from build123d import *

# Parameters (mm, degrees)
F2_DEPTH = 5
F1_R     = 1.5
F3_DEPTH = 5


with BuildPart() as f2:
    # F0 (on Top) → F2 (new body)
    with BuildSketch(Plane.XY):
        with BuildLine():
            add(Edge.make_bspline(
                [(28.7786647677, 16.4962057024), (27.3534332712, 16.4962057024), (25.9282017748, 16.3979139179), (24.5029702783, 16.3979139179)],
                knots=[0, 0, 0, 0, 4.2768241304, 4.2768241304, 4.2768241304, 4.2768241304], degree=3))
            add(Edge.make_bspline(
                [(28.7786647677, 16.4962057024), (30.1958868901, 16.5288864324), (31.6131090124, 16.5615671625), (33.0303311348, 16.5942478925)],
                knots=[0, 0, 0, 0, 4.252796629, 4.252796629, 4.252796629, 4.252796629], degree=3))
            add(Edge.make_bspline(
                [(34.0554304421, 15.8441737294), (33.7053959568, 16.1608718336), (33.3803656201, 16.2775497884), (33.0303311348, 16.5942478925)],
                knots=[0, 0, 0, 0, 1.2702125176, 1.2702125176, 1.2702125176, 1.2702125176], degree=3))
            add(Edge.make_bspline(
                [(35.030528903, 7.8683812171), (34.7054960827, 10.5269787212), (34.3804632624, 13.1855762253), (34.0554304421, 15.8441737294)],
                knots=[0, 0, 0, 0, 8.0351778579, 8.0351778579, 8.0351778579, 8.0351778579], degree=3))
            add(Edge.make_bspline(
                [(36.1056365073, 5.4181381129), (35.9264295305, 5.3620166626), (35.3451776861, 5.1799886127), (35.15918074, 6.7691662645), (35.030528903, 7.8683812171)],
                knots=[0, 0, 0, 0, 0.3083121001, 1, 1, 1, 1], degree=3))
            add(Edge.make_bspline(
                [(38.8059057295, 8.4184361622), (37.4535769802, 6.9203687349), (36.1012482309, 5.4223013077), (36.1056365073, 5.4181381129)],
                knots=[0, 0, 0, 0, 0.9144176852, 0.9144176852, 0.9144176852, 0.9144176852], degree=3))
            add(Edge.make_bspline(
                [(39.8560129106, 14.1940098256), (39.2937416175, 11.3257224468), (38.7314703243, 8.4574350679), (38.8059057295, 8.4184361622)],
                knots=[0, 0, 0, 0, 0.9279806118, 0.9279806118, 0.9279806118, 0.9279806118], degree=3))
            add(Edge.make_bspline(
                [(43.4063635767, 19.4445308298), (41.6661026772, 16.796114764), (39.8167199055, 13.9816315759), (39.8538236249, 14.1821767609), (39.8560129106, 14.1940098256)],
                knots=[0, 0, 0, 0, 0.9409955181, 1, 1, 1, 1], degree=3))
            add(Edge.make_bspline(
                [(46.1316332221, 30.1705934107), (46.201065216, 26.0141822855), (46.2669693032, 19.7845163706), (44.1314354539, 19.7195578367), (43.4063635767, 19.4445308298)],
                knots=[0, 0, 0, 0, 0.6856364339, 1, 1, 1, 1], degree=3))
            add(Edge.make_bspline(
                [(44.0814308822, 39.2214953899), (44.942471716, 37.026856873), (45.9936424251, 33.4912353698), (46.1571893395, 30.7073156698), (46.1316332221, 30.1705934107)],
                knots=[0, 0, 0, 0, 0.5973818248, 1, 1, 1, 1], degree=3))
            add(Edge.make_bspline(
                [(37.9308201373, 46.5972237289), (39.7218772443, 45.1967775697), (42.7448053753, 42.833118659), (43.922661607, 39.3325250293), (44.0814308822, 39.2214953899)],
                knots=[0, 0, 0, 0, 0.5634229372, 0.9509395541, 0.9509395541, 0.9509395541, 0.9509395541], degree=3))
            add(Edge.make_bspline(
                [(28.3798743039, 49.4475066662), (30.3463351664, 49.2764352977), (34.0485912428, 48.954359214), (36.6916346322, 47.3496080436), (37.9308201373, 46.5972237289)],
                knots=[0, 0, 0, 0, 0.5311520386, 1, 1, 1, 1], degree=3))
            add(Edge.make_bspline(
                [(20.4540863633, 47.2972951829), (21.8867810289, 47.9304252414), (24.6135730188, 49.1354370372), (27.1677144968, 49.3470690664), (28.3798743039, 49.4475066662)],
                knots=[0, 0, 0, 0, 0.5254139923, 1, 1, 1, 1], degree=3))
            add(Edge.make_bspline(
                [(12.128260918, 36.621235311), (13.2656434176, 39.1604577253), (15.3840794859, 43.8898960188), (18.8493227012, 46.2187817818), (20.4540863633, 47.2972951829)],
                knots=[0, 0, 0, 0, 0.5368972501, 1, 1, 1, 1], degree=3))
            add(Edge.make_bspline(
                [(11.1531633884, 25.0700879842), (11.0426565419, 27.5454372876), (10.8424476096, 32.0301100206), (11.730414239, 35.2006838689), (12.128260918, 36.621235311)],
                knots=[0, 0, 0, 0, 0.5519576234, 1, 1, 1, 1], degree=3))
            add(Edge.make_bspline(
                [(12.128260918, 20.2196072787), (11.9396298399, 20.7302181813), (11.4960442281, 21.93097286), (11.2783087006, 23.9243676733), (11.1531633884, 25.0700879842)],
                knots=[0, 0, 0, 0, 0.4252416515, 1, 1, 1, 1], degree=3))
            add(Edge.make_bspline(
                [(14.2806209624, 19.1009379923), (13.5631676142, 19.4738277545), (12.8457142661, 19.8467175166), (12.128260918, 20.2196072787)],
                knots=[0, 0, 0, 0, 2.4257111809, 2.4257111809, 2.4257111809, 2.4257111809], degree=3))
            add(Edge.make_bspline(
                [(17.6962614059, 13.7686077505), (16.5577145914, 15.5460511645), (15.4191677769, 17.3234945784), (14.2806209624, 19.1009379923)],
                knots=[0, 0, 0, 0, 6.3324833555, 6.3324833555, 6.3324833555, 6.3324833555], degree=3))
            add(Edge.make_bspline(
                [(18.826616928, 7.7482336201), (18.449831754, 9.7550249969), (18.07304658, 11.7618163737), (17.6962614059, 13.7686077505)],
                knots=[0, 0, 0, 0, 6.1255700369, 6.1255700369, 6.1255700369, 6.1255700369], degree=3))
            add(Edge.make_bspline(
                [(21.8245182186, 5.4629491642), (21.7108202341, 5.3376502894), (21.4165861788, 5.0133947963), (20.4957638936, 6.0671498654), (19.4532904711, 7.1170784645), (18.826616928, 7.7482336201)],
                knots=[0, 0, 0, 0, 0.2007630192, 0.5195458611, 1, 1, 1, 1], degree=3))
            add(Edge.make_bspline(
                [(22.9794476181, 12.7365430817), (22.5944711516, 10.3120117759), (22.2094946851, 7.88748047), (21.8245182186, 5.4629491642)],
                knots=[0, 0, 0, 0, 7.3647152283, 7.3647152283, 7.3647152283, 7.3647152283], degree=3))
            add(Edge.make_bspline(
                [(24.5029702783, 16.3979139179), (24.2545480757, 16.457738394), (23.7733196994, 16.5750358032), (23.1531511766, 15.0702995523), (23.0738569515, 13.5969865217), (22.9794476181, 12.7365430817)],
                knots=[0, 0, 0, 0, 0.2229298737, 0.552268584, 1, 1, 1, 1], degree=3))
        make_face()
        with BuildLine():
            add(Edge.make_bspline(
                [(19.7707619518, 25.4675038159), (20.2849085132, 25.757982706), (20.6410096337, 26.1077272395), (21.1551561952, 26.3982061297)],
                knots=[0, 0, 0, 0, 1.6681589307, 1.6681589307, 1.6681589307, 1.6681589307], degree=3))
            add(Edge.make_bspline(
                [(21.1551561952, 26.3982061297), (21.8123979867, 26.8640990059), (22.4696397781, 27.329991882), (23.1268815696, 27.7958847582)],
                knots=[0, 0, 0, 0, 2.4168588087, 2.4168588087, 2.4168588087, 2.4168588087], degree=3))
            add(Edge.make_bspline(
                [(23.1268815696, 27.7958847582), (23.4302642999, 27.9257749489), (23.9764650926, 28.1596251916), (24.333578659, 27.9078247286), (24.4923364371, 27.7958847582)],
                knots=[0, 0, 0, 0, 0.5554417612, 1, 1, 1, 1], degree=3))
            add(Edge.make_bspline(
                [(24.4923364371, 27.7958847582), (24.7112412104, 27.5568410681), (25.0480976986, 27.1889942788), (25.0461675905, 26.9821026564), (25.045491755, 26.9096586853)],
                knots=[0, 0, 0, 0, 0.6498457975, 1, 1, 1, 1], degree=3))
            add(Edge.make_bspline(
                [(25.045491755, 26.9096586853), (25.0901061339, 26.6330206678), (25.1757880791, 26.0779728274), (24.7261609493, 25.6500168981), (24.4923364371, 25.4675038159)],
                knots=[0, 0, 0, 0, 0.4901555982, 1, 1, 1, 1], degree=3))
            add(Edge.make_bspline(
                [(24.4923364371, 25.4675038159), (23.2477368166, 24.5850893358), (22.0031371961, 23.7619404991), (20.7585375756, 22.8795260191)],
                knots=[0, 0, 0, 0, 4.5430037437, 4.5430037437, 4.5430037437, 4.5430037437], degree=3))
            add(Edge.make_bspline(
                [(20.7585375756, 22.8795260191), (20.405901409, 22.8403885896), (19.7724884957, 22.7700890696), (19.4290917953, 23.0786102264), (19.2768722773, 23.2153702527)],
                knots=[0, 0, 0, 0, 0.5567239935, 1, 1, 1, 1], degree=3))
            add(Edge.make_bspline(
                [(19.2768722773, 23.2153702527), (19.1175545535, 23.4298293637), (18.8164909813, 23.845577707), (18.8726020293, 24.2868788492), (18.9015176147, 24.5192367584)],
                knots=[0, 0, 0, 0, 0.5178862764, 1, 1, 1, 1], degree=3))
            add(Edge.make_bspline(
                [(18.9015176147, 24.5192367584), (18.9318202689, 24.6817342211), (19.1368350812, 25.0158121965), (19.5525943822, 25.3099724303), (19.7707619518, 25.4675038159)],
                knots=[0, 0, 0, 0, 0.4488819495, 1, 1, 1, 1], degree=3))
        make_face(mode=Mode.SUBTRACT)
        with BuildLine():
            add(Edge.make_bspline(
                [(32.6592810452, 25.869358331), (32.4509113562, 26.0499476175), (32.2939669471, 26.3610240009), (32.1994835702, 26.8554791141), (32.5083631343, 27.4777518027), (32.8954510162, 27.8253639918), (33.5004289129, 27.9999233062), (33.9412095353, 27.9802175247), (34.1260544956, 27.8949011117)],
                knots=[0, 0, 0, 0, 0.1726951713, 0.3215696796, 0.4991474643, 0.6559863652, 0.8270618313, 1, 1, 1, 1], degree=3))
            add(Edge.make_bspline(
                [(34.1260544956, 27.8949011117), (35.4740905265, 26.8984256933), (36.8221265574, 25.9019502749), (38.1701625884, 24.9054748565)],
                knots=[0, 0, 0, 0, 5.0290634915, 5.0290634915, 5.0290634915, 5.0290634915], degree=3))
            add(Edge.make_bspline(
                [(38.1701625884, 24.9054748565), (38.2405595194, 24.8143368767), (38.4020654987, 24.6052463887), (38.470948132, 23.977433478), (38.2329838854, 23.2694437637), (37.6073773996, 22.8025261291), (37.0741936096, 22.8121444764), (36.8011705577, 22.8170696646)],
                knots=[0, 0, 0, 0, 0.1512568335, 0.3470163066, 0.5621197723, 0.7757782618, 1, 1, 1, 1], degree=3))
            add(Edge.make_bspline(
                [(36.8011705577, 22.8170696646), (35.4205407202, 23.8344992201), (34.0399108827, 24.8519287755), (32.6592810452, 25.869358331)],
                knots=[0, 0, 0, 0, 5.1450670391, 5.1450670391, 5.1450670391, 5.1450670391], degree=3))
        make_face(mode=Mode.SUBTRACT)
    extrude(amount=F2_DEPTH)

    # F1 (on face) → F3 (cut)
    with BuildSketch(Plane.XY):
        with Locations((23.01017569, 32.86326798)):
            Circle(F1_R)
        with Locations((-15598.762805792, 35.025678575)):
            Circle(F1_R)
        with Locations((34.2861823738, 32.8629463911)):
            Circle(F1_R)
        with Locations((23.0116825551, 37.5390388072)):
            Circle(F1_R)
        with Locations((28.6087393761, 37.5647246838)):
            Circle(F1_R)
        with Locations((34.2885330319, 37.5625342131)):
            Circle(F1_R)
        with Locations((23.0116825551, 42.2612205148)):
            Circle(F1_R)
        with Locations((28.6087393761, 42.23600775)):
            Circle(F1_R)
        with Locations((34.265037626, 42.2377288342)):
            Circle(F1_R)
        with Locations((28.6087393761, 32.8614637256)):
            Circle(F1_R)
    extrude(amount=F3_DEPTH, mode=Mode.SUBTRACT)


solid = f2.part
Geometry check sheet. Reference: the model listing, model coordinates, mm. Give positions to 0.01 mm unless a question says otherwise; leave off trailing zeros.
1) Cross-section at A-A (x = 22.5). Give the number of separate pieces and of enclosed holes in the cut face, then the cut area to 3 significant figures.
Results are:
separate pieces: 5
enclosed holes: 0
area: 134 mm2
2) Material ranges on probe 1 along Y at (x, z) = (35.5, 1.6); probe 2 along Y at (x, z) = (33, 0.75); probe 3 along X at (y, z) = (15, 2.55), recorded low to high.
Results are:
probe 1: y = 5.54 to 23.78, 26.88 to 31.98, 33.74 to 36.68, 38.45 to 41.39, 43.09 to 47.96
probe 2: y = 16.59 to 25.62, 27.83 to 32.09, 33.63 to 36.79, 38.33 to 41.43, 43.04 to 48.84
probe 3: x = 16.91 to 23.26, 34.16 to 40.46
3) Draft check along Y on faces 1 (the flat face through (29, 28, 0)), 2 (the cylindrical face through (27.418, 31.949, 2.465)). Enter one of: released by +Y, released by -Y, zero draft, split by the parting line, or undercut.
Results are:
face 1: zero draft
face 2: undercut
4) Gauge pin test, flat ends, axial feed: pin 1 (1 mm diameter, centred on y = 22, z = 1, fed in from +X); pin 2 (1 mm diameter, centred on x = 41.5, z = 2.5, fed in from -Y); pin 3 (1 mm diameter, centred on y = 32.5, z = 1, fed in from +X). Record the tip position at first contact, or that the pin passes through.
Results are:
pin 1: stops at x = 45.92
pin 2: stops at y = 15.8
pin 3: stops at x = 46.03
